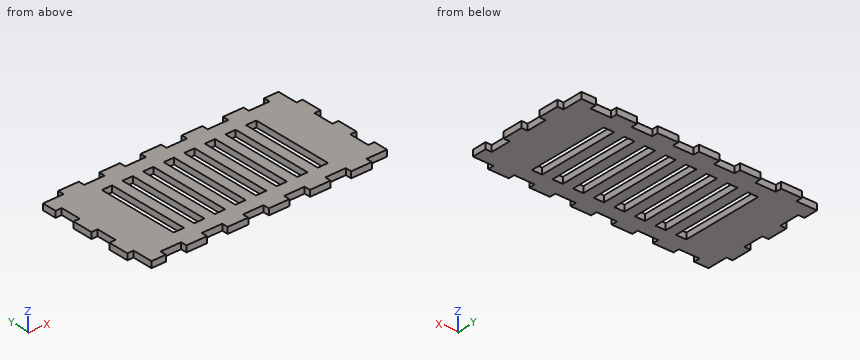
```python
from build123d import *

# Parameters (mm, degrees)
BOSS_EXTRUDE1_DEPTH = 3
SKETCH2_W           = 5
SKETCH2_H           = 40
CUT_EXTRUDE1_DEPTH  = 10


with BuildPart() as part:
    # Sketch1 → Boss-Extrude1 (new body)
    with BuildSketch(Plane.XY):
        Polygon((120, 3), (120, 10), (117, 10), (117, 20), (120, 20), (120, 30), (117, 30), (117, 40), (120, 40), (120, 50), (117, 50), (117, 60), (110, 60), (110, 57), (100, 57), (100, 60), (90, 60), (90, 57), (80, 57), (80, 60), (70, 60), (70, 57), (60, 57), (60, 60), (50, 60), (50, 57), (40, 57), (40, 60), (30, 60), (30, 57), (20, 57), (20, 60), (10, 60), (10, 57), (0, 57), (0, 50), (3, 50), (3, 40), (0, 40), (0, 30), (3, 30), (3, 20), (0, 20), (0, 10), (3, 10), (3, 0), (10, 0), (10, 3), (20, 3), (20, 0), (30, 0), (30, 3), (40, 3), (40, 0), (50, 0), (50, 3), (60, 3), (60, 0), (70, 0), (70, 3), (80, 3), (80, 0), (90, 0), (90, 3), (100, 3), (100, 0), (110, 0), (110, 3), align=None)
    extrude(amount=BOSS_EXTRUDE1_DEPTH)

    # Sketch2 → Cut-Extrude1 (cut)
    with BuildSketch(Plane.XY.offset(3)):
        with Locations((25, 30)):
            Rectangle(SKETCH2_W, SKETCH2_H)
        with Locations((35, 30)):
            Rectangle(SKETCH2_W, SKETCH2_H)
        with Locations((45, 30)):
            Rectangle(SKETCH2_W, SKETCH2_H)
        with Locations((55, 30)):
            Rectangle(SKETCH2_W, SKETCH2_H)
        with Locations((65, 30)):
            Rectangle(SKETCH2_W, SKETCH2_H)
        with Locations((75, 30)):
            Rectangle(SKETCH2_W, SKETCH2_H)
        with Locations((85, 30)):
            Rectangle(SKETCH2_W, SKETCH2_H)
        with Locations((95, 30)):
            Rectangle(SKETCH2_W, SKETCH2_H)
    extrude(amount=-CUT_EXTRUDE1_DEPTH, mode=Mode.SUBTRACT)


solid = part.part
```
The model under review builds one solid part; all positions refer to its coordinate system, in mm. Coordinates: 2 decimals unless noted, no trailing zeros. Write each loop counter-clockwise with the first axis right and the second up, starting at its lowest first coordinate (ties: lowest second). Pieces come first, ordered by that corner, then holes.
1) We need section A-A on y = 25. Count the separate pieces of the cut face and the enclosed holes in it, then the cut area to 3 significant figures.
2) Clearance check with flat-ended pins moving along their axes: pin 1 Ø1 at (x, z) = (74, 1) entering from -Y; pin 2 Ø1.5 at (x, z) = (104, 1.5) entering from +Y; pin 3 Ø1.5 at (y, z) = (58, 2) entering from -X. State where each tip first meets the part, or that it passes through.
3) We need section C-C on x = 113. State the section outline as (y, z) points.
4) To check wall thickness, follow probe 1 along Y at (x, z) = (43, 0.5); probe 2 along Y at (x, z) = (82, 0.8); probe 3 along Y at (x, z) = (56.5, 1). State the ranges of each line that lie inside material, in increasing order.
Answer list:
1. separate pieces: 9
1. enclosed holes: 0
1. area: 231 mm2
2. pin 1: stops at y = 3
2. pin 2: stops at y = 57
2. pin 3: stops at x = 10
3. outline: (3, 0) - (60, 0) - (60, 3) - (3, 3) - close
4. probe 1: y = 0 to 10, 50 to 57
4. probe 2: y = 0 to 57
4. probe 3: y = 3 to 10, 50 to 60
